from build123d import *

# Parameters (mm, degrees)
SKETCH1_W               = 152.4
SKETCH1_H               = 190.5
BOSS_EXTRUDE1_DEPTH     = 25.4
SKETCH2_R               = 26.67
CUT_EXTRUDE1_DEPTH      = 125.595997127
CUT_EXTRUDE3_DEPTH      = 125.595997127
CUT_EXTRUDE3_DEPTH_BACK = 125.595997127
SKETCH3_R               = 3.175
CUT_EXTRUDE4_DEPTH      = 125.595997127
CUT_EXTRUDE4_DEPTH_BACK = 125.595997127
SKETCH4_R               = 44.45
CUT_EXTRUDE5_DEPTH      = 125.595997127
CUT_EXTRUDE5_DEPTH_BACK = 125.595997127
SKETCH6_R               = 3.175
CUT_EXTRUDE6_DEPTH      = 125.595997127
CUT_EXTRUDE6_DEPTH_BACK = 125.595997127
SKETCH7_R               = 3.175
SKETCH8_R               = 3.175
CUT_EXTRUDE7_DEPTH      = 25.4


with BuildPart() as part:
    # Sketch1 → Boss-Extrude1 (new body)
    with BuildSketch(Plane.XY):
        Rectangle(SKETCH1_W, SKETCH1_H)
    extrude(amount=BOSS_EXTRUDE1_DEPTH)

    # Sketch2 → Cut-Extrude1 (cut, through all)
    with BuildSketch(Plane(origin=(0, 0, 0), x_dir=(-1, 0, 0), z_dir=(0, 0, -1))):
        with Locations((0, 57.15)):
            Circle(SKETCH2_R)
    extrude(amount=-CUT_EXTRUDE1_DEPTH, mode=Mode.SUBTRACT)

    # Sketch3 → Cut-Extrude3 (cut, two sides: drawn at the far end of the back side and taken through both)
    with BuildSketch(Plane(origin=(0, 0, 0), x_dir=(-1, 0, 0), z_dir=(0, 0, -1)).offset(-CUT_EXTRUDE3_DEPTH_BACK)):
        with Locations((-63.5, 82.55)):
            Circle(SKETCH3_R)
        with Locations((63.5, 82.55)):
            Circle(SKETCH3_R)
        with Locations((63.5, -82.55)):
            Circle(SKETCH3_R)
        with Locations((-63.5, -82.55)):
            Circle(SKETCH3_R)
    extrude(amount=CUT_EXTRUDE3_DEPTH + CUT_EXTRUDE3_DEPTH_BACK, mode=Mode.SUBTRACT)

    # Sketch4 → Cut-Extrude4 (cut, two sides: drawn at the far end of the back side and taken through both)
    with BuildSketch(Plane(origin=(0, 0, 0), x_dir=(-1, 0, 0), z_dir=(0, 0, -1)).offset(-CUT_EXTRUDE4_DEPTH_BACK)):
        with Locations((0, -25.4)):
            Circle(SKETCH4_R)
    extrude(amount=CUT_EXTRUDE4_DEPTH + CUT_EXTRUDE4_DEPTH_BACK, mode=Mode.SUBTRACT)

    # Sketch6 → Cut-Extrude5 (cut, two sides: drawn at the far end of the back side and taken through both)
    with BuildSketch(Plane(origin=(0, 0, 0), x_dir=(-1, 0, 0), z_dir=(0, 0, -1)).offset(-CUT_EXTRUDE5_DEPTH_BACK)):
        with Locations((-63.5, 19.05)):
            Circle(SKETCH6_R)
        with Locations((63.5, 19.05)):
            Circle(SKETCH6_R)
    extrude(amount=CUT_EXTRUDE5_DEPTH + CUT_EXTRUDE5_DEPTH_BACK, mode=Mode.SUBTRACT)

    # Sketch7 → Cut-Extrude6 (cut, two sides: drawn at the far end of the back side and taken through both)
    with BuildSketch(Plane(origin=(0, 0, 0), x_dir=(-1, 0, 0), z_dir=(0, 0, -1)).offset(-CUT_EXTRUDE6_DEPTH_BACK)):
        with Locations((-57.15, -63.5)):
            Circle(SKETCH7_R)
        with Locations((57.15, -63.5)):
            Circle(SKETCH7_R)
    extrude(amount=CUT_EXTRUDE6_DEPTH + CUT_EXTRUDE6_DEPTH_BACK, mode=Mode.SUBTRACT)

    # Sketch8 → Cut-Extrude7 (cut)
    with BuildSketch(Plane(origin=(0, 95.25, 0), x_dir=(1, 0, 0), z_dir=(0, 1, 0))):
        with Locations(Location((0, -12.7, 0), (0, 0, 180))):
            Circle(SKETCH8_R)
    extrude(amount=-CUT_EXTRUDE7_DEPTH, mode=Mode.SUBTRACT)


solid = part.part
Model file for the job. Use its own axes, mm. A direction names the side the tool comes from. Coordinates: 2 decimals unless noted, no trailing zeros. Loops run counter-clockwise (first coordinate to the right, second up) from the corner with the lowest first, then second, coordinate; pieces in that order, holes last. Notation, with made-up numbers: (74, -36) -> (104, -36) arc R22 cw to (104, -18) -> close; hole circle Ø9 at (69, -27.75). An arc over 180 degrees is marked (long way). Use one line per item in the form item = value. Start each with the question number.
(1) Cut at B-B on x = 57.15. Give the cut face in (y, z) (3 decimals).
(2) Cut at C-C on z = 22. Give the number of separate pieces and of enclosed holes in the cut face, and give its area (3 significant figures).
(3) Flat gauge pin, fed straight in: pin 1 (5 mm diameter, centred on x = -63.5, y = -82.55, fed in from -Z). Where does the tip first touch, or does it go through?
(4) Cut at A-A on y = 57.15. Give the cut face in (x, z).
(5) Cut at D-D on y = -63.5. Give the cut face in (x, z) (3 decimals).
(6) Probe probe 1 along X at (y, z) = (-82, 19.5); probe 2 along X at (y, z) = (-82.55, 6.25) (3 decimals); probe 3 along Y at (x, z) = (63.5, 8) (3 decimals). List the from-to ranges inside material, lowest first. Write a range as from..to.
(7) Tool access for faces 1 (the cylindrical face through (-1.5, 89.5, 9.9)), 2 (the cylindrical face through (-66.53, -81.6, 12.88)): list every direction of +Z, -Z, +X, -X, +Y, -Y with a clear straight run to the whole face (end or side of a thin tool).
(8) Pull direction X, two halves, no side cores. Call faces 3 (the cylindrical face through (5.79, 18.67, 12.88)), 4 (the flat face through (-76.2, -1, 13)), 5 (the flat face through (-1, 23, 0)), 6 (the flat face through (76.2, -1, 13)): pulls with the +X half, pulls with the -X half, needs draft (parallel to the pull), parting line crosses it, or undercut.
Values:
q1.outline = (-95.25, 0) -> (-66.675, 0) -> (-66.675, 25.4) -> (-95.25, 25.4) -> close; (-60.325, 0) -> (95.25, 0) -> (95.25, 25.4) -> (-60.325, 25.4) -> close
q2.separate_pieces = 1
q2.enclosed_holes = 10
q2.area = 20,300 mm2
q3.pin_1 = through
q4.outline = (-76.2, 0) -> (-26.67, 0) -> (-26.67, 25.4) -> (-76.2, 25.4) -> close; (26.67, 0) -> (76.2, 0) -> (76.2, 25.4) -> (26.67, 25.4) -> close
q5.outline = (-76.2, 0) -> (-60.325, 0) -> (-60.325, 25.4) -> (-76.2, 25.4) -> close; (-53.975, 0) -> (-22.895, 0) -> (-22.895, 25.4) -> (-53.975, 25.4) -> close; (22.895, 0) -> (53.975, 0) -> (53.975, 25.4) -> (22.895, 25.4) -> close; (60.325, 0) -> (76.2, 0) -> (76.2, 25.4) -> (60.325, 25.4) -> close
q6.probe_1 = -76.2..-66.63, -60.37..60.37, 66.63..76.2
q6.probe_2 = -76.2..-66.675, -60.325..60.325, 66.675..76.2
q6.probe_3 = -95.25..-85.725, -79.375..15.875, 22.225..79.375, 85.725..95.25
q7.face_1 = +Y
q7.face_2 = +Z, -Z
q8.face_3 = undercut
q8.face_4 = pulls with the -X half
q8.face_5 = needs draft
q8.face_6 = pulls with the +X half
